Autodesk Inventor part; units mm, degrees
ref_plane "YZ Plane" through (0, 0, 0) normal (1, 0, 0) x (0, 1, 0)
ref_plane "XZ Plane" through (0, 0, 0) normal (0, 1, 0) x (-1, 0, 0)
ref_plane "XY Plane" through (0, 0, 0) normal (0, 0, 1) x (1, 0, 0)
sketch "Esquisse1" plane through (0, 0, 0) normal (1, 0, 0) x (0, 1, 0)
  line L0 (0, 0) -> (28, 0)
  line L1 (28, 0) -> (28, -17)
  line L2 (28, -17) -> (0, -17)
  line L3 (0, -17) -> (0, 0)
  line L4 (0, 0) -> (0, -2)
  line L5 (0, -2) -> (2, -2)
  line L6 (28, -17) -> (28, -15)
  line L7 (28, -15) -> (26, -15)
  line L8 (26, -15) -> (2, -15)
  line L9 (2, -15) -> (2, -2)
  line L10 (2, -2) -> (26, -2)
  line L11 (26, -2) -> (26, -15)
  dimension "d1" = 28
  dimension "d2" = 17
  dimension "d3" = 2
  dimension "d4" = 2
  dimension "d5" = 2
  dimension "d6" = 2
extrude "Extrusion1" add sketch "Esquisse1" along normal blind 13.5 contours L0 L1 L7 L11 L10 L5 L3 | L5 L9 L8 L7 L1 L2 L3
sketch "Esquisse2" plane through (0, 0, 0) normal (-1, 0, 0) x (0, 0, 1)
  line L0 (-2, 2) -> (-2, 26)
  line L1 (-2, 26) -> (-15, 26)
  line L2 (-15, 26) -> (-15, 2)
  line L3 (-15, 2) -> (-2, 2)
  line L4 (-2, 2) -> (-2, 26)
  point P0 (0, 0)
extrude "Extrusion2" add sketch "Esquisse2" against normal blind 2
sketch "Esquisse3" plane through (2, 0, 0) normal (1, 0, 0) x (0, 0, -1)
  line L0 (15, 2) -> (2, 2)
  line L1 (2, 2) -> (2, 19.4)
  line L2 (2, 2) -> (2, 26)
  line L3 (2, 19.4) -> (2, 21.5)
  line L4 (2, 21.5) -> (2, 26)
  line L5 (2, 21.5) -> (2, 26)
  line L6 (15, 2) -> (2, 2)
  line L7 (2, 2) -> (2, 19.4)
  line L8 (2, 19.4) -> (15, 19.4)
  line L9 (15, 19.4) -> (15, 2)
  line L10 (2, 26) -> (15, 26)
  line L11 (15, 26) -> (2, 26)
  line L12 (2, 26) -> (2, 21.5)
  line L13 (2, 21.5) -> (15, 21.5)
  line L14 (15, 21.5) -> (15, 26)
  point P0 (0, 0)
  dimension "d11" = 17.4
  dimension "d12" = 2.1
extrude "Extrusion3" add sketch "Esquisse3" along normal blind 4.5
sketch "Esquisse4" plane through (6.5, 0, 0) normal (1, 0, 0) x (0, 0, -1)
  line L0 (15, 2) -> (2, 2)
  line L1 (15, 2) -> (2, 2)
  line L2 (2, 2) -> (2, 8)
  line L3 (2, 8) -> (15, 8)
  line L4 (15, 8) -> (15, 2)
  point P0 (0, 0)
  dimension "d15" = 6
extrude "Extrusion4" cut sketch "Esquisse4" against normal blind 2
sketch "Esquisse5" plane through (13.5, 26, -15) normal (0, -1, 0) x (1, 0, 0)
  line L0 (-9, 13) -> (0, 13)
  line L1 (-9, 0) -> (0, 0)
  arc A0 (0, 13) -> (0, 0) centre (-0.4821, 6.5) ccw
  line L2 (0, 0) -> (0, 13)
  line L3 (0, 13) -> (0, 0)
  point P0 (-13.5, 15)
extrude "Extrusion5" cut sketch "Esquisse5" against normal up to next
fillet "Congé1" radius 1 1 edges at (0, 14, 0)
fillet "Congé2" radius 1 1 edges at (0, 14, -17)
fillet "Congé3" radius 1 5 edges at (0.2929, 28, -0.2929) (7.25, 28, 0) (0.2929, 28, -16.7071) (7.25, 28, -17) (0, 28, -8.5)
fillet "Congé4" radius 1 5 edges at (0.2929, 0, -16.7071) (7.25, 0, -17) (0.2929, 0, -0.2929) (7.25, 0, 0) (0, 0, -8.5)
properties part number "Support servomoteur"
Here's how the part is built. I have some questions about the finished solid (model axes, mm). A direction names the side the tool comes from. Round coordinates to 2 decimals unless told otherwise and drop trailing zeros. Loops run counter-clockwise (first coordinate to the right, second up) from the corner with the lowest first, then second, coordinate; pieces in that order, holes last.
1. If we section it at C-C on y = 22.25: Write out the boundary of the cut face in (x, z), plus the area to 3 significant figures.
Answer list:
outline: (0, -16) arc R1 ccw to (1, -17) - (13.5, -17) - (13.5, -15) - (6.5, -15) - (6.5, -2) - (13.5, -2) - (13.5, 0) - (1, 0) arc R1 ccw to (0, -1) - close
area: 138 mm2
2. If we section it at A-A on x = 3.25: Write out the boundary of the cut face in (y, z).
Answer list:
outline: (0, -16) arc R1 ccw to (1, -17) - (27, -17) arc R1 ccw to (28, -16) - (28, -1) arc R1 ccw to (27, 0) - (1, 0) arc R1 ccw to (0, -1) - close; hole (19.4, -15) - (21.5, -15) - (21.5, -2) - (19.4, -2) - close
3. If we section it at B-B on x = 5.5: Write out the boundary of the cut face in (y, z).
Answer list:
outline: (0, -16) arc R1 ccw to (1, -17) - (27, -17) arc R1 ccw to (28, -16) - (28, -1) arc R1 ccw to (27, 0) - (1, 0) arc R1 ccw to (0, -1) - close; hole (2, -15) - (8, -15) - (8, -2) - (2, -2) - close; hole (19.4, -15) - (21.5, -15) - (21.5, -2) - (19.4, -2) - close
4. For P1, Ø1.8, axis at y = 4, z = -6, coming from the +X side; P2, Ø3, axis at x = 9.5, z = -8.5, coming from the -Y side; P3, Ø5, axis at y = 24.5, z = -5.5, coming from the +X side; P4, Ø1.1, axis at y = 20, z = -9.5, coming from the +X side, each with a flat end and sliding along its axis, tell me the tip position at first contact or that it passes through.
Answer list:
P1: stops at x = 4.5
P2: stops at y = 0
P3: stops at x = 8.84
P4: stops at x = 2
5. We'd pull the mould along Y, two halves only. Please class faces 1 (the face through (0.285, 14.182, -0.301)), 2 (the face through (4, 21.5, -8)), 3 (the face through (6, 28, -8)), 4 (the face through (6.5, 14, -8)): +Y half, -Y half, draft (parallel to the pull), parting line (faces both ways), or undercut.
Answer list:
face 1: draft
face 2: undercut
face 3: +Y half
face 4: undercut
6. If I drill on line 1 along Y through (x, z) = (5.5, -2.25); line 2 along Y through (x, z) = (4, -13.75); line 3 along Z through (x, y) = (13, 17.5), over which ranges is the centre line in solid material (lowest first)?
Answer list:
line 1: y = 0 to 2, 8 to 19.4, 21.5 to 28
line 2: y = 0 to 19.4, 21.5 to 28
line 3: z = -17 to -15, -2 to 0
7. Which directions (+Z, -Z, +X, -X, +Y, -Y) give clear straight access to the entire face, cutting with the end or side of a thin tool? Please do faces 5 (the face through (7.162, 27.715, -16.699)), 6 (the face through (4.5, 5, -8)).
Answer list:
face 5: -Z, +X, -X, +Y
face 6: +X
8. If we section it at D-D on z = -14.5: Write out the boundary of the cut face in (x, y).
Answer list:
outline: (0, 1) arc R1 ccw to (1, 0) - (13.5, 0) - (13.5, 2) - (4.5, 2) - (4.5, 8) - (6.5, 8) - (6.5, 19.4) - (2, 19.4) - (2, 21.5) - (6.5, 21.5) - (6.5, 26) - (10.47, 26) - (10.47, 28) - (1, 28) arc R1 ccw to (0, 27) - close
